from build123d import *

# Parameters (mm, degrees)
SKETCH_1_W          = 130
SKETCH_1_H          = 130
EXTRUDE_1_DEPTH     = 3
SKETCH_2_R          = 2.6
CUT_EXTRUDE_1_DEPTH = 92.972822073
SKETCH_4_W          = 20.650518397
SKETCH_4_H          = 20.951555191
CUT_EXTRUDE_2_DEPTH = 1
SKETCH_5_W          = 88.698963206
SKETCH_5_H          = 5.1
SKETCH_5_W_2        = 5.1
SKETCH_5_H_2        = 88.096889618
CUT_EXTRUDE_3_DEPTH = 1
CUT_EXTRUDE_4_DEPTH = 3
EXTRUDE_START       = -2
SKETCH_7_R          = 1.25
EXTRUDE_2_DEPTH     = 2
FILLET_1_R          = 1
SKETCH_15_R         = 8.25
CUT_EXTRUDE_9_DEPTH = 92.972822073
CHAMFER_1_SIZE      = 1
CHAMFER_2_SIZE      = 0.2
FILLET_3_R          = 1
FILLET_4_R          = 1


with BuildPart() as part:
    # 草图1 → 凸台-拉伸1 (new body)
    with BuildSketch(Plane(origin=(0, 0, 0), x_dir=(1, 0, 0), z_dir=(0, 1, 0))):
        Rectangle(SKETCH_1_W, SKETCH_1_H)
    extrude(amount=EXTRUDE_1_DEPTH)

    # 草图2 → 切除-拉伸1 (cut, through all)
    with BuildSketch(Plane(origin=(0, 3, 0), x_dir=(1, 0, 0), z_dir=(0, 1, 0))):
        with Locations(Location((52.5, 52.5, 0), (0, 0, 270))):
            Circle(SKETCH_2_R)
        with Locations(Location((52.5, -52.5, 0), (0, 0, 270))):
            Circle(SKETCH_2_R)
        with Locations(Location((-52.5, -52.5, 0), (0, 0, 270))):
            Circle(SKETCH_2_R)
        with Locations(Location((-52.5, 52.5, 0), (0, 0, 270))):
            Circle(SKETCH_2_R)
    extrude(amount=-CUT_EXTRUDE_1_DEPTH, mode=Mode.SUBTRACT)

    # 草图4 → 切除-拉伸2 (cut)
    with BuildSketch(Plane(origin=(0, 3, 0), x_dir=(1, 0, 0), z_dir=(0, 1, 0))):
        with Locations((54.674740802, 54.524222405)):
            Rectangle(SKETCH_4_W, SKETCH_4_H)
        with Locations((-54.674740802, -54.524222405)):
            Rectangle(SKETCH_4_W, SKETCH_4_H)
        with Locations((54.674740802, -54.524222405)):
            Rectangle(SKETCH_4_W, SKETCH_4_H)
        with Locations((-54.674740802, 54.524222405)):
            Rectangle(SKETCH_4_W, SKETCH_4_H)
    extrude(amount=-CUT_EXTRUDE_2_DEPTH, mode=Mode.SUBTRACT)

    # 草图5 → 切除-拉伸3 (cut)
    with BuildSketch(Plane(origin=(0, 3, 0), x_dir=(1, 0, 0), z_dir=(0, 1, 0))):
        with Locations((0, 62.45)):
            Rectangle(SKETCH_5_W, SKETCH_5_H)
        with Locations((62.45, 0)):
            Rectangle(SKETCH_5_W_2, SKETCH_5_H_2)
        with Locations((0, -62.45)):
            Rectangle(SKETCH_5_W, SKETCH_5_H)
        with Locations((-62.45, 0)):
            Rectangle(SKETCH_5_W_2, SKETCH_5_H_2)
    extrude(amount=-CUT_EXTRUDE_3_DEPTH, mode=Mode.SUBTRACT)

    # 草图6 → 切除-拉伸4 (cut)
    with BuildSketch(Plane(origin=(0, 0, 0), x_dir=(-1, 0, 0), z_dir=(0, -1, 0))):
        with BuildLine():
            Line((47.5, -35), (47.5, 35))
            ThreePointArc((47.5, 35), (46.035533906, 38.535533906), (42.5, 40))
            Line((42.5, 40), (21.5, 40))
            ThreePointArc((21.5, 40), (17.964466094, 38.535533906), (16.5, 35))
            Line((16.5, 35), (16.5, -35))
            ThreePointArc((16.5, -35), (17.964466094, -38.535533906), (21.5, -40))
            Line((21.5, -40), (42.5, -40))
            ThreePointArc((42.5, -40), (46.035533906, -38.535533906), (47.5, -35))
        make_face()
    extrude(amount=-CUT_EXTRUDE_4_DEPTH, mode=Mode.SUBTRACT)

    # 草图7 → 凸台-拉伸2 (add)
    # profile 1 of 4: a face of its own
    with BuildSketch(Plane(origin=(0, 3, 0), x_dir=(1, 0, 0), z_dir=(0, 1, 0)).offset(EXTRUDE_START)):
        with BuildLine():
            Line((-24.75, 40), (-24.75, 31.75))
            Line((-24.75, 31.75), (-16.5, 31.75))
            Line((-16.5, 31.75), (-16.5, 35))
            ThreePointArc((-16.5, 35), (-17.964466094, 38.535533906), (-21.5, 40))
            Line((-21.5, 40), (-24.75, 40))
        make_face()
        with Locations(Location((-20.872307757, 35.627692243, 0), (0, 0, 270))):
            Circle(SKETCH_7_R, mode=Mode.SUBTRACT)
    # profile 2 of 4: a face of its own
    with BuildSketch(Plane(origin=(0, 3, 0), x_dir=(1, 0, 0), z_dir=(0, 1, 0)).offset(EXTRUDE_START)):
        with BuildLine():
            Line((-16.5, -31.75), (-24.75, -31.75))
            Line((-24.75, -31.75), (-24.75, -40))
            Line((-24.75, -40), (-21.5, -40))
            ThreePointArc((-21.5, -40), (-17.964466094, -38.535533906), (-16.5, -35))
            Line((-16.5, -35), (-16.5, -31.75))
        make_face()
        with Locations(Location((-20.872307757, -35.627692243, 0), (0, 0, 270))):
            Circle(SKETCH_7_R, mode=Mode.SUBTRACT)
    # profile 3 of 4: a face of its own
    with BuildSketch(Plane(origin=(0, 3, 0), x_dir=(1, 0, 0), z_dir=(0, 1, 0)).offset(EXTRUDE_START)):
        with BuildLine():
            Line((-39.25, -40), (-39.25, -31.75))
            Line((-39.25, -31.75), (-47.5, -31.75))
            Line((-47.5, -31.75), (-47.5, -35))
            ThreePointArc((-47.5, -35), (-46.035533906, -38.535533906), (-42.5, -40))
            Line((-42.5, -40), (-39.25, -40))
        make_face()
        with Locations(Location((-43.127692243, -35.627692243, 0), (0, 0, 270))):
            Circle(SKETCH_7_R, mode=Mode.SUBTRACT)
    # profile 4 of 4: a face of its own
    with BuildSketch(Plane(origin=(0, 3, 0), x_dir=(1, 0, 0), z_dir=(0, 1, 0)).offset(EXTRUDE_START)):
        with BuildLine():
            Line((-47.5, 31.75), (-39.25, 31.75))
            Line((-39.25, 31.75), (-39.25, 40))
            Line((-39.25, 40), (-42.5, 40))
            ThreePointArc((-42.5, 40), (-46.035533906, 38.535533906), (-47.5, 35))
            Line((-47.5, 35), (-47.5, 31.75))
        make_face()
        with Locations(Location((-43.127692243, 35.627692243, 0), (0, 0, 270))):
            Circle(SKETCH_7_R, mode=Mode.SUBTRACT)
    extrude(amount=EXTRUDE_2_DEPTH)

    # 圆角1
    fillet_1_edges = [part.edges().sort_by_distance(p)[0] for p in [
        (-24.75, 2, -31.75),
        (-39.25, 2, -31.75),
        (-39.25, 2, 31.75),
        (-24.75, 2, 31.75),
    ]]
    fillet(fillet_1_edges, radius=FILLET_1_R)

    # 草图15 → 切除-拉伸9 (cut, through all)
    with BuildSketch(Plane(origin=(0, 0, 0), x_dir=(-1, 0, 0), z_dir=(0, -1, 0))):
        with Locations(Location((-37, -37, 0), (0, 0, 90))):
            Circle(SKETCH_15_R)
    extrude(amount=-CUT_EXTRUDE_9_DEPTH, mode=Mode.SUBTRACT)

    # 倒角1
    chamfer_1_edges = [part.edges().sort_by_distance(p)[0] for p in [
        (0, 0, 65),
        (-65, 0, 0),
        (0, 0, -65),
        (65, 0, 0),
    ]]
    chamfer(chamfer_1_edges, length=CHAMFER_1_SIZE)

    # 倒角2
    chamfer_2_edges = [part.edges().sort_by_distance(p)[0] for p in [
        (65, 1.5, 65),
        (-65, 1.5, 65),
        (-65, 1.5, -65),
        (65, 1.5, -65),
    ]]
    chamfer(chamfer_2_edges, length=CHAMFER_2_SIZE)

    # 圆角3
    fillet_3_edges = [part.edges().sort_by_distance(p)[0] for p in [
        (59.9, 2.5, 44.048444809),
        (59.9, 2.5, -44.048444809),
        (-44.349481603, 2.5, -59.9),
        (44.349481603, 2.5, -59.9),
        (44.349481603, 2.5, 59.9),
        (-44.349481603, 2.5, 59.9),
        (-59.9, 2.5, 44.048444809),
        (-59.9, 2.5, -44.048444809),
        (-44.349481603, 2.5, -44.048444809),
        (-44.349481603, 2.5, 44.048444809),
        (44.349481603, 2.5, 44.048444809),
        (44.349481603, 2.5, -44.048444809),
    ]]
    fillet(fillet_3_edges, radius=FILLET_3_R)

    # 圆角4
    fillet_4_edges = [part.edges().sort_by_distance(p)[0] for p in [
        (-24.75, 2, -40),
        (-16.5, 2, -31.75),
        (-47.5, 2, -31.75),
        (-39.25, 2, -40),
        (-39.25, 2, 40),
        (-47.5, 2, 31.75),
        (-16.5, 2, 31.75),
        (-24.75, 2, 40),
    ]]
    fillet(fillet_4_edges, radius=FILLET_4_R)


solid = part.part
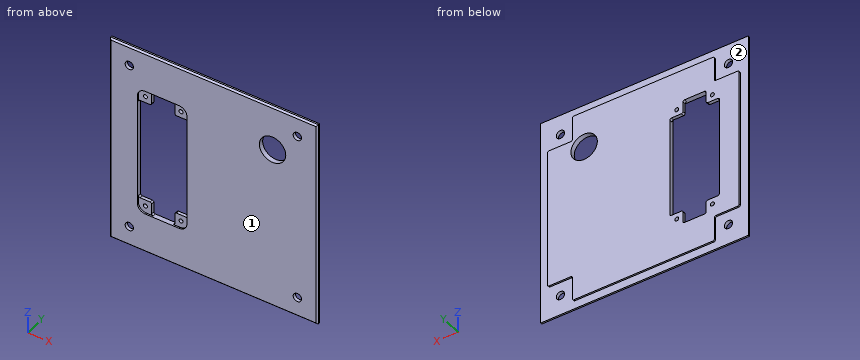
Input: part model. Units: mm. Frame: model coordinates. Face numbers are marked on the shaded views. A direction names the side the tool comes from. Coordinates: 2 decimals unless noted, no trailing zeros. Loops run counter-clockwise (first coordinate to the right, second up) from the corner with the lowest first, then second, coordinate; pieces in that order, holes last. Notation, with made-up numbers: (12.5, 19.5) -> (26.5, 19.5) arc R31 ccw to (26.5, 48.5) -> close; hole circle Ø2 at (-29, 51). An arc over 180 degrees is marked (long way). One line per item, written item: value.
(1) Cut plane D-D (x = 37). Output: boundary loops of the cut face in (y, z).
Answer below:
outline: (0, -64) -> (1, -65) -> (2, -65) -> (2, -59.9) -> (3, -59.9) -> (3, 28.75) -> (0, 28.75) -> close; (0, 45.25) -> (3, 45.25) -> (3, 59.9) -> (2, 59.9) -> (2, 65) -> (1, 65) -> (0, 64) -> close
(2) Cut plane C-C (z = -18). Output: boundary loops of the cut face in (x, y).
Answer below:
outline: (-65, 1) -> (-64, 0) -> (-47.5, 0) -> (-47.5, 3) -> (-59.9, 3) -> (-59.9, 2) -> (-65, 2) -> close; (-16.5, 0) -> (64, 0) -> (65, 1) -> (65, 2) -> (59.9, 2) -> (59.9, 3) -> (-16.5, 3) -> close
(3) Pin query (flat end, axial travel): pin 1 Ø4.5 at (x, z) = (-42, -33) entering from -Y; pin 2 Ø0.8 at (y, z) = (2.5, -49.5) entering from -X; pin 3 Ø0.5 at (y, z) = (2.5, 3) entering from -X; pin 4 Ø7 at (x, z) = (52.5, -52.5) entering from -Y. Return the tip coordinate at first contact, or that it passes through.
Answer below:
pin 1: stops at y = 1
pin 2: stops at x = -44.35
pin 3: stops at x = -59.9
pin 4: stops at y = 0
(4) Ray query, line 1 along X through (y, z) = (0.8, -52.5); line 2 along X through (y, z) = (1.45, 20.5); line 3 along Z through (x, y) = (-29.5, 1). Return the intervals inside material, ascending.
Answer below:
line 1: x = -64.8 to -55.1, -49.9 to 49.9, 55.1 to 64.8
line 2: x = -65 to -47.5, -16.5 to 65
line 3: z = -65 to -40, 40 to 65
(5) Cut plane A-A (x = 52.5). Output: boundary loops of the cut face in (y, z), then the cut area to 3 significant figures.
Answer below:
outline: (0, -64) -> (1, -65) -> (2, -65) -> (2, -55.1) -> (0, -55.1) -> close; (0, -49.9) -> (2, -49.9) -> (2, -44.05) -> (3, -44.05) -> (3, 44.05) -> (2, 44.05) -> (2, 49.9) -> (0, 49.9) -> close; (0, 55.1) -> (2, 55.1) -> (2, 65) -> (1, 65) -> (0, 64) -> close
area: 326 mm2
(6) Set-up query: the marked faces 1 and 2. Return all of +Z, -Z, +X, -X, +Y, -Y with unobstructed straight access to the full face (end or side cutting, diameter ignored); none if empty.
Answer below:
face 1: +Z, -Z, +X, -X, -Y
face 2: +Y
(7) Cut plane B-B (z = -52.5). Output: boundary loops of the cut face in (x, y), then the cut area to 3 significant figures.
Answer below:
outline: (-65, 1) -> (-64, 0) -> (-55.1, 0) -> (-55.1, 2) -> (-65, 2) -> close; (-49.9, 0) -> (49.9, 0) -> (49.9, 2) -> (44.35, 2) -> (44.35, 3) -> (-44.35, 3) -> (-44.35, 2) -> (-49.9, 2) -> close; (55.1, 0) -> (64, 0) -> (65, 1) -> (65, 2) -> (55.1, 2) -> close
area: 327 mm2
